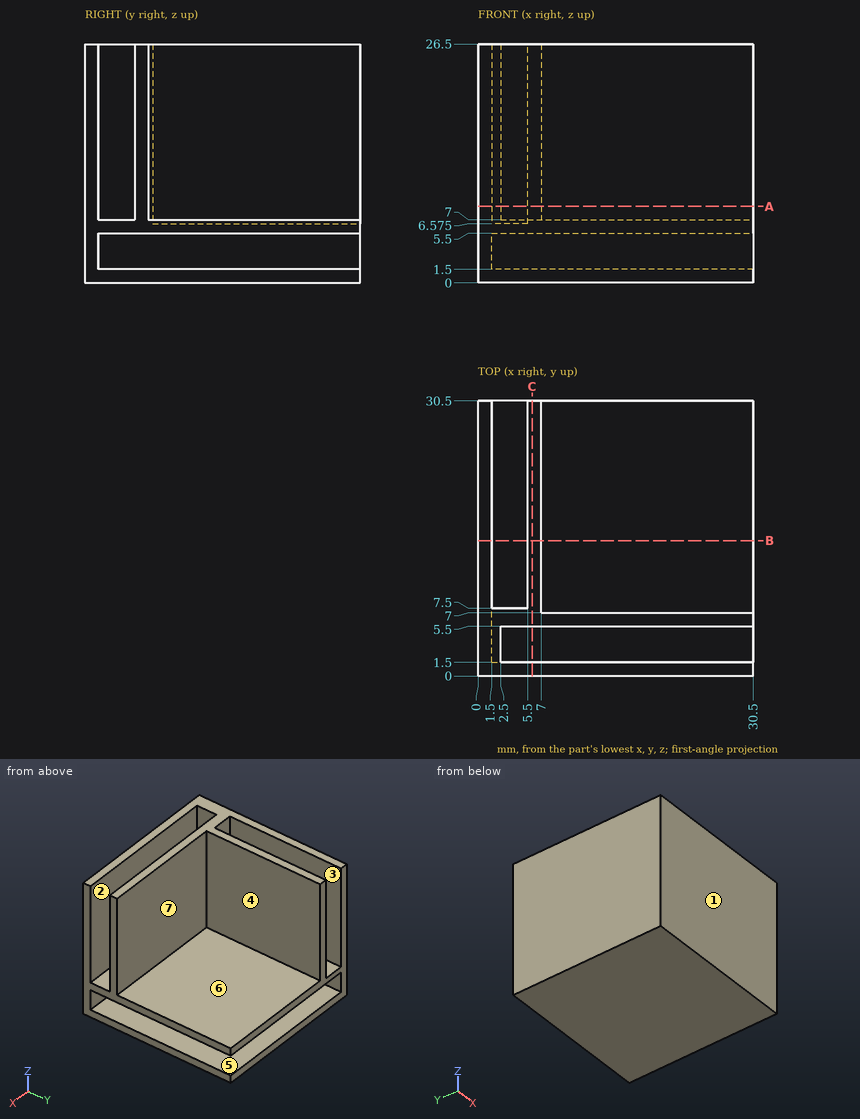
Part print with two shaded views. Sizes in mm from the minimum x, y, z corner. A direction names the side the tool comes from. Give positions to 0.01 mm unless a question says otherwise; leave off trailing zeros. Loops run counter-clockwise (first coordinate to the right, second up) from the corner with the lowest first, then second, coordinate; pieces in that order, holes last. Notation, with made-up numbers: (24.25, -12.75) - (81.25, -12.75) arc R26 cw to (81.25, 6.25) - close; hole circle Ø9 at (46.5, 31.25). An arc over 180 degrees is marked (long way). Put each result on its own line as item: value.
Q1. Slice it at A-A (z = 8.5). Give the cut face in (x, y), plus the area to 3 significant figures.
Filled in:
outline: (0, 0) - (30.5, 0) - (30.5, 1.5) - (2.5, 1.5) - (2.5, 5.5) - (30.5, 5.5) - (30.5, 7) - (7, 7) - (7, 30.5) - (5.5, 30.5) - (5.5, 7.5) - (1.5, 7.5) - (1.5, 30.5) - (0, 30.5) - close
area: 174 mm²
Q2. Mould opens along Z. For the marked faces 5, 6 and 7 say: pulls with the +Z half, pulls with the -Z half, needs draft (parallel to the pull), parting line crosses it, or undercut.
Filled in:
face 5: undercut
face 6: pulls with the +Z half
face 7: needs draft
Q3. Flat gauge pins, fed straight in: pin 1 (2 mm diameter, centred on y = 4, z = 21, fed in from +X); pin 2 (12 mm diameter, centred on y = 14.5, z = 20, fed in from +X); pin 3 (1.2 mm diameter, centred on x = 13.5, y = 3, fed in from +Z). Where does each tip first touch, or does it go through?
Filled in:
pin 1: stops at x = 2.5
pin 2: stops at x = 7
pin 3: stops at z = 7
Q4. Slice it at C-C (x = 6). Give the cut face in (y, z), plus the area to 3 significant figures.
Filled in:
outline: (0, 0) - (30.5, 0) - (30.5, 1.5) - (1.5, 1.5) - (1.5, 5.5) - (30.5, 5.5) - (30.5, 26.5) - (5.5, 26.5) - (5.5, 7) - (1.5, 7) - (1.5, 26.5) - (0, 26.5) - close
area: 614 mm²
Q5. Tool access for the marked faces 1, 2, 3 and 4: list every direction of +Z, -Z, +X, -X, +Y, -Y with a clear straight run to the whole face (end or side of a thin tool).
Filled in:
face 1: +Z, -Z, +X, -X, -Y
face 2: +Z, +X
face 3: +Z, +Y
face 4: +Z, +X, +Y
Q6. Probe line 1 along X through (y, z) = (12, 12.25). List the from-to ranges inside material, lowest first.
Filled in:
line 1: x = 0 to 1.5, 5.5 to 7
Q7. Slice it at B-B (y = 15). Give the cut face in (x, z) (3 decimals).
Filled in:
outline: (0, 0) - (30.5, 0) - (30.5, 1.5) - (1.5, 1.5) - (1.5, 5.5) - (30.5, 5.5) - (30.5, 7) - (7, 7) - (7, 26.5) - (5.5, 26.5) - (5.5, 6.575) - (1.5, 6.575) - (1.5, 26.5) - (0, 26.5) - close
